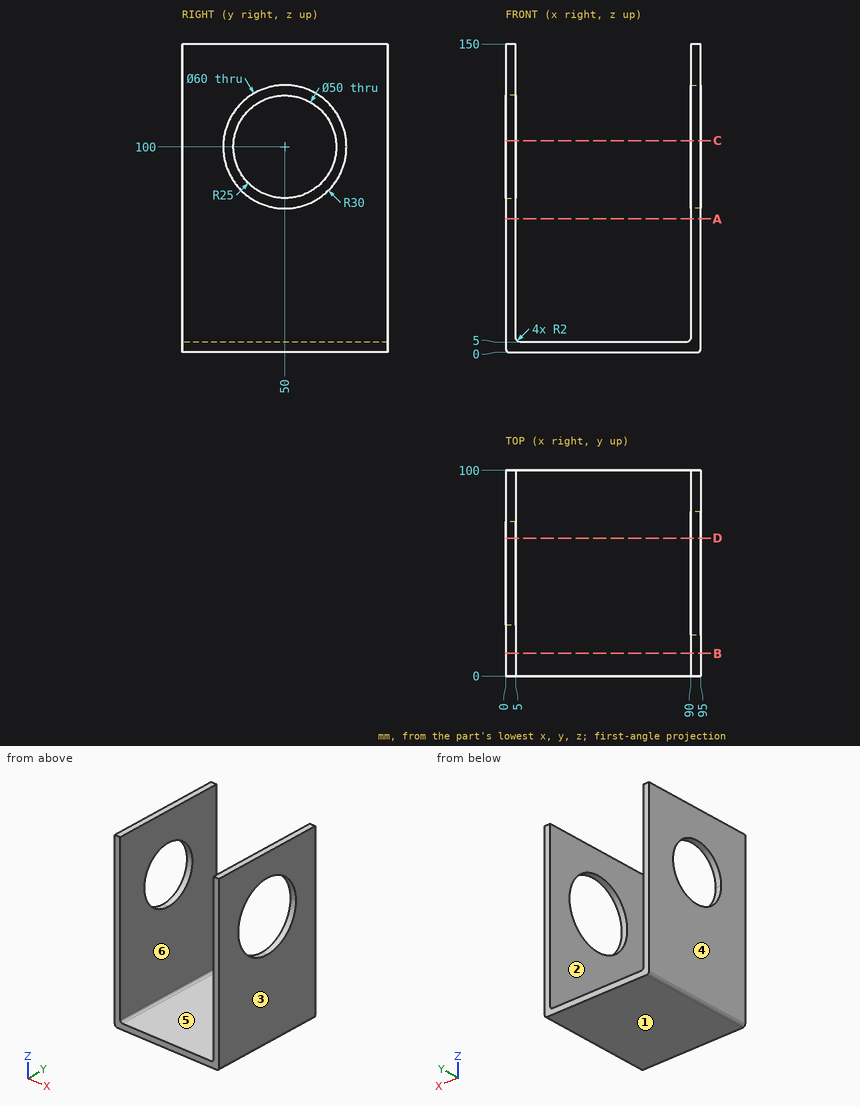
For this review, use the dimensioned drawing (mm, ordinates from the lowest corner) and the shaded views. A direction names the side the tool comes from. Give positions to 0.01 mm unless a question says otherwise; leave off trailing zeros. Loops run counter-clockwise (first coordinate to the right, second up) from the corner with the lowest first, then second, coordinate; pieces in that order, holes last. Notation, with made-up numbers: (69, 47.25) -> (122, 47.25) arc R19 cw to (122, 64.25) -> close; hole circle Ø2 at (54.25, -36). An arc over 180 degrees is marked (long way). One line per question, with ' | ' between items. Start each with the question number.
(1) We need section D-D (y = 67). State the section outline as (x, z) points, and give its area (3 significant figures).
(2) For the marked faces 1 and 2, list the 3-axis set-ups (+Z, -Z, +X, -X, +Y, -Y) from which the entire face can be reached by the end or side of a thin tool; tool diameter is ignored.
(3) For line 1 (Y direction, x = 1.65, z = 100); line 2 (Z direction, x = 93.4, y = 50); line 3 (X direction, y = 46, z = 24.5), list the stretches that pass through material, from the lowest coordinate up.
(4) Insertion check: P1, Ø3, axis at x = 35.5, y = 77.5, coming from the +Z side; P2, Ø2, axis at y = 77, z = 84.5, coming from the -X side. Each pin has a flat end and moves straight along its axis. Give the tip position at first contact, or say it passes through.
(5) We need section A-A (z = 65). State the section outline as (x, y) points, and give its area (4 significant figures).
(6) We need section B-B (y = 11). State the section outline as (x, z) points, and give its area (4 significant figures).
(7) Draft analysis for pull direction X (two halves, no side actions). For the marked faces 3, 4, 5 and 6, state which applies: +X half, -X half, draft (parallel to the pull), parting line (faces both ways), or undercut.
(8) We need section C-C (z = 103). State the section outline as (x, y) points, and give its area (3 significant figures).
The answers:
1) outline: (0, 2) arc R2 ccw to (2, 0) -> (93, 0) arc R2 ccw to (95, 2) -> (95, 75.28) -> (90, 75.28) -> (90, 7) arc R2 cw to (88, 5) -> (7, 5) arc R2 cw to (5, 7) -> (5, 81.67) -> (0, 81.67) -> close; (0, 118.33) -> (5, 118.33) -> (5, 150) -> (0, 150) -> close; (90, 124.72) -> (95, 124.72) -> (95, 150) -> (90, 150) -> close | area: 1,490 mm^2
2) face 1: -Z, +X, -X, +Y, -Y | face 2: +Z, +Y, -Y
3) line 1: y = 0 to 25, 75 to 100 | line 2: z = 0.04 to 70, 130 to 150 | line 3: x = 0 to 5, 90 to 95
4) P1: stops at z = 5 | P2: stops at x = 0
5) outline: (0, 0) -> (5, 0) -> (5, 100) -> (0, 100) -> close; (90, 0) -> (95, 0) -> (95, 100) -> (90, 100) -> close | area: 1,000 mm^2
6) outline: (0, 2) arc R2 ccw to (2, 0) -> (93, 0) arc R2 ccw to (95, 2) -> (95, 150) -> (90, 150) -> (90, 7) arc R2 cw to (88, 5) -> (7, 5) arc R2 cw to (5, 7) -> (5, 150) -> (0, 150) -> close | area: 1,925 mm^2
7) face 3: +X half | face 4: -X half | face 5: undercut | face 6: undercut
8) outline: (0, 0) -> (5, 0) -> (5, 25.18) -> (0, 25.18) -> close; (0, 74.82) -> (5, 74.82) -> (5, 100) -> (0, 100) -> close; (90, 0) -> (95, 0) -> (95, 20.15) -> (90, 20.15) -> close; (90, 79.85) -> (95, 79.85) -> (95, 100) -> (90, 100) -> close | area: 453 mm^2
